Work out the finished part from the listing and answer in its coordinate system (mm). Face numbers are marked on the shaded views. A direction names the side the tool comes from. Give positions to 0.01 mm unless a question says otherwise; leave off trailing zeros. Write each loop counter-clockwise with the first axis right and the second up, starting at its lowest first coordinate (ties: lowest second). Pieces come first, ordered by that corner, then holes.
1) Find section C-C (y = 5.5). Determine the outline of the cut face in (x, z).
2) Given pin 1 Ø2.5 at (y, z) = (14.5, -2.5) entering from -X; pin 2 Ø1 at (y, z) = (2, -4) entering from +X, each flat-ended and moving along its own axis, determine where each tip first touches the part or whether it passes through.
3) Straight lines are drawn through the part: probe 1 along X at (y, z) = (3.5, -3.6); probe 2 along Y at (x, z) = (3, -3.8); probe 3 along X at (y, z) = (5.75, -4). For each, find the intervals that lie inside material, in ascending order.
4) Find section D-D (y = 16.5). Determine the outline of the cut face in (x, z).
5) Determine the mould class of the marked faces 3, 4 and 5 for opening direction Y: pulls with the +Y half, pulls with the -Y half, needs draft (parallel to the pull), parting line crosses it, or undercut.
6) Find section A-A (z = -1.1). Determine the outline of the cut face in (x, y), plus the area to 3 significant figures.
7) Find section B-B (x = 43). Determine the outline of the cut face in (y, z).
8) A tool of negligible diameter and unlimited length cuts with its end or side. For the marked faces 1 and 2, from which of +Z, -Z, +X, -X, +Y, -Y can it reach the whole face along a straight path? Write none if from no direction.
```python
from build123d import *

# Parameters (mm, degrees)
SKETCH_1_W          = 46
SKETCH_1_H          = 20
SKETCH_1_R          = 1.7
EXTRUDE_1_DEPTH     = 5
SKETCH_3_W          = 41
SKETCH_3_H          = 10
CUT_EXTRUDE_1_DEPTH = 5
FILLET_1_R          = 3
SKETCH_4_W          = 4
SKETCH_4_H          = 20
EXTRUDE_2_DEPTH     = 5
FILLET_2_R          = 3
FILLET_3_R          = 3


with BuildPart() as part:
    # 草图1 → 凸台-拉伸1 (new body)
    with BuildSketch(Plane.XY):
        with Locations((23, 10)):
            Rectangle(SKETCH_1_W, SKETCH_1_H)
        with Locations((3, 5)):
            Circle(SKETCH_1_R, mode=Mode.SUBTRACT)
        with Locations((43, 5)):
            Circle(SKETCH_1_R, mode=Mode.SUBTRACT)
    extrude(amount=-EXTRUDE_1_DEPTH)

    # 草图3 → 切除-拉伸1 (cut)
    with BuildSketch(Plane.XY):
        with Locations((20.5, 15)):
            Rectangle(SKETCH_3_W, SKETCH_3_H)
    extrude(amount=-CUT_EXTRUDE_1_DEPTH, mode=Mode.SUBTRACT)

    # 圆角1
    fillet_1_edges = [part.edges().sort_by_distance(p)[0] for p in [
        (0, 10, -2.5),
        (41, 20, -2.5),
    ]]
    fillet(fillet_1_edges, radius=FILLET_1_R)

    # 草图4 → 凸台-拉伸2 (add)
    with BuildSketch(Plane.XY):
        with Locations((48, 10)):
            Rectangle(SKETCH_4_W, SKETCH_4_H)
    extrude(amount=-EXTRUDE_2_DEPTH)

    # 圆角2
    fillet_2_edges = [part.edges().sort_by_distance(p)[0] for p in [
        (50, 20, -2.5),
        (50, 0, -2.5),
    ]]
    fillet(fillet_2_edges, radius=FILLET_2_R)

    # 圆角3
    fillet_3_edges = [part.edges().sort_by_distance(p)[0] for p in [
        (0, 0, -2.5),
    ]]
    fillet(fillet_3_edges, radius=FILLET_3_R)


solid = part.part
```
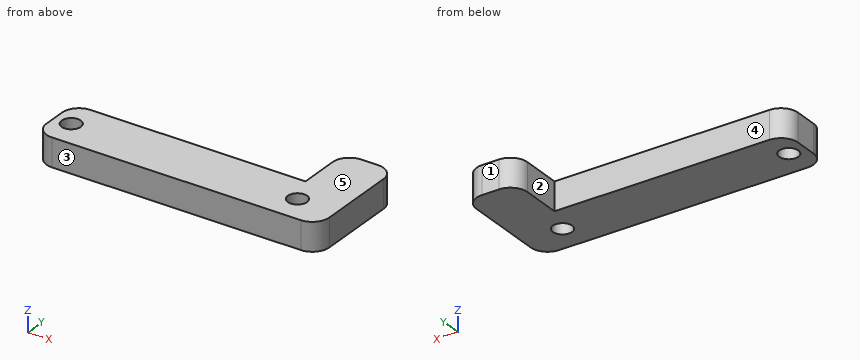
Results:
1. outline: (0, -5) - (1.38, -5) - (1.38, 0) - (0, 0) - close; (4.62, -5) - (41.38, -5) - (41.38, 0) - (4.62, 0) - close; (44.62, -5) - (50, -5) - (50, 0) - (44.62, 0) - close
2. pin 1: stops at x = 41
2. pin 2: stops at x = 49.96
3. probe 1: x = 0 to 2.2, 3.8 to 42.2, 43.8 to 50
3. probe 2: y = 0 to 3.3, 6.7 to 10
3. probe 3: x = 0 to 1.47, 4.53 to 41.47, 44.53 to 50
4. outline: (41, -5) - (50, -5) - (50, 0) - (41, 0) - close
5. face 3: pulls with the -Y half
5. face 4: pulls with the +Y half
5. face 5: needs draft
6. outline: (0, 3) arc R3 ccw to (3, 0) - (47, 0) arc R3 ccw to (50, 3) - (50, 17) arc R3 ccw to (47, 20) - (44, 20) arc R3 ccw to (41, 17) - (41, 10) - (3, 10) arc R3 ccw to (0, 7) - close; hole circle Ø3.4 at (3, 5); hole circle Ø3.4 at (43, 5)
6. area: 562 mm2
7. outline: (0, -5) - (3.3, -5) - (3.3, 0) - (0, 0) - close; (6.7, -5) - (19.83, -5) - (19.83, 0) - (6.7, 0) - close
8. face 1: +Z, -Z, +X, -X, +Y
8. face 2: +Z, -Z, -X, +Y
